Geometry: final body of the model. Coordinates: model frame, mm. Give positions to 0.01 mm unless a question says otherwise; leave off trailing zeros. Write item = value, one per line. Start each with the question number.
from build123d import *

# Parameters (mm, degrees)
CHAMFER1_SIZE                   = 3
FILLET3_R                       = 5
SKETCH3_R                       = 6
CUT_EXTRUDE3_DEPTH              = 152.492574214
CIRPATTERN2_COUNT               = 5
CIRPATTERN2_ANGLE               = 60
CIRPATTERN2_THE_OTHER_WAY_COUNT = 5
CIRPATTERN2_THE_OTHER_WAY_ANGLE = 60
MIRROR1_COPY_1_SKETCH_R         = 6
MIRROR1_COPY_1_DEPTH            = 152.492574214
MIRROR1_COPY_2_SKETCH_R         = 6
MIRROR1_COPY_2_DEPTH            = 152.492574214
MIRROR1_COPY_3_SKETCH_R         = 6
MIRROR1_COPY_3_DEPTH            = 152.492574214
MIRROR1_COPY_4_SKETCH_R         = 6
MIRROR1_COPY_4_DEPTH            = 152.492574214
MIRROR1_COPY_5_SKETCH_R         = 6
MIRROR1_COPY_5_DEPTH            = 152.492574214
MIRROR1_COPY_6_SKETCH_R         = 6
MIRROR1_COPY_6_DEPTH            = 152.492574214
MIRROR1_COPY_7_SKETCH_R         = 6
MIRROR1_COPY_7_DEPTH            = 152.492574214
MIRROR1_COPY_8_SKETCH_R         = 6
MIRROR1_COPY_8_DEPTH            = 152.492574214


with BuildPart() as part:
    # Sketch1 → Revolve1 (revolve)
    with BuildSketch(Plane.XY, mode=Mode.PRIVATE) as revolve1_sk:
        Polygon((15, 105), (7.442388155, 105), (0, 97.557611845), (-7.442388155, 105), (-15, 105), (-15, 73), (15, 73), align=None)
    revolve(revolve1_sk.sketch.rotate(Axis((0, 0, 0), (1, 0, 0)), 90), axis=Axis((0, 0, 0), (1, 0, 0)))

    # Chamfer1
    chamfer1_edges = [part.edges().sort_by_distance(p)[0] for p in [
        (15, 0, -73),
        (-15, 0, -73),
    ]]
    chamfer(chamfer1_edges, length=CHAMFER1_SIZE)

    # Fillet3
    fillet3_edges = [part.edges().sort_by_distance(p)[0] for p in [
        (0, 0, -97.557611845),
    ]]
    fillet(fillet3_edges, radius=FILLET3_R)

    # Sketch3 → Cut-Extrude3 (cut, through all)
    with BuildSketch(Plane(origin=(15, 0, 0), x_dir=(0, 0, -1), z_dir=(1, 0, 0))):
        with Locations((0, 85)):
            Circle(SKETCH3_R)
    cut_extrude3 = extrude(amount=-CUT_EXTRUDE3_DEPTH, mode=Mode.SUBTRACT)

    # CirPattern2: Cut-Extrude3 ×5 about axis
    cirpattern2_axis = Axis((0, 0, 0), (-1, 0, 0))
    for i in range(1, CIRPATTERN2_COUNT):
        add(cut_extrude3.rotate(cirpattern2_axis, i * CIRPATTERN2_ANGLE / (CIRPATTERN2_COUNT - 1)), mode=Mode.SUBTRACT)

    # CirPattern2 the other way: Cut-Extrude3 ×5 about axis
    cirpattern2_the_other_way_axis = Axis((0, 0, 0), (1, 0, 0))
    for i in range(1, CIRPATTERN2_THE_OTHER_WAY_COUNT):
        add(cut_extrude3.rotate(cirpattern2_the_other_way_axis, i * CIRPATTERN2_THE_OTHER_WAY_ANGLE / (CIRPATTERN2_THE_OTHER_WAY_COUNT - 1)), mode=Mode.SUBTRACT)

    # Mirror1: Cut-Extrude3 across plane
    add(cut_extrude3.mirror(Plane.ZX), mode=Mode.SUBTRACT)

    # Mirror1 copy 1 sketch → Mirror1 copy 1 (cut, through all)
    with BuildSketch(Plane(origin=(15, 0, 0), x_dir=(0, 0.2588190451025214, -0.9659258262890681), z_dir=(1, 0, 0))):
        with Locations((0, -85)):
            Circle(MIRROR1_COPY_1_SKETCH_R)
    extrude(amount=-MIRROR1_COPY_1_DEPTH, mode=Mode.SUBTRACT)

    # Mirror1 copy 2 sketch → Mirror1 copy 2 (cut, through all)
    with BuildSketch(Plane(origin=(15, 0, 0), x_dir=(0, 0.5000000000000011, -0.866025403784438), z_dir=(1, 0, 0))):
        with Locations((0, -85)):
            Circle(MIRROR1_COPY_2_SKETCH_R)
    extrude(amount=-MIRROR1_COPY_2_DEPTH, mode=Mode.SUBTRACT)

    # Mirror1 copy 3 sketch → Mirror1 copy 3 (cut, through all)
    with BuildSketch(Plane(origin=(15, 0, 0), x_dir=(0, 0.7071067811865488, -0.7071067811865462), z_dir=(1, 0, 0))):
        with Locations((0, -85)):
            Circle(MIRROR1_COPY_3_SKETCH_R)
    extrude(amount=-MIRROR1_COPY_3_DEPTH, mode=Mode.SUBTRACT)

    # Mirror1 copy 4 sketch → Mirror1 copy 4 (cut, through all)
    with BuildSketch(Plane(origin=(15, 0, 0), x_dir=(0, 0.8660254037844399, -0.4999999999999978), z_dir=(1, 0, 0))):
        with Locations((0, -85)):
            Circle(MIRROR1_COPY_4_SKETCH_R)
    extrude(amount=-MIRROR1_COPY_4_DEPTH, mode=Mode.SUBTRACT)

    # Mirror1 copy 5 sketch → Mirror1 copy 5 (cut, through all)
    with BuildSketch(Plane(origin=(15, 0, 0), x_dir=(0, -0.2588190451025214, -0.9659258262890681), z_dir=(1, 0, 0))):
        with Locations((0, -85)):
            Circle(MIRROR1_COPY_5_SKETCH_R)
    extrude(amount=-MIRROR1_COPY_5_DEPTH, mode=Mode.SUBTRACT)

    # Mirror1 copy 6 sketch → Mirror1 copy 6 (cut, through all)
    with BuildSketch(Plane(origin=(15, 0, 0), x_dir=(0, -0.5000000000000011, -0.866025403784438), z_dir=(1, 0, 0))):
        with Locations((0, -85)):
            Circle(MIRROR1_COPY_6_SKETCH_R)
    extrude(amount=-MIRROR1_COPY_6_DEPTH, mode=Mode.SUBTRACT)

    # Mirror1 copy 7 sketch → Mirror1 copy 7 (cut, through all)
    with BuildSketch(Plane(origin=(15, 0, 0), x_dir=(0, -0.7071067811865488, -0.7071067811865462), z_dir=(1, 0, 0))):
        with Locations((0, -85)):
            Circle(MIRROR1_COPY_7_SKETCH_R)
    extrude(amount=-MIRROR1_COPY_7_DEPTH, mode=Mode.SUBTRACT)

    # Mirror1 copy 8 sketch → Mirror1 copy 8 (cut, through all)
    with BuildSketch(Plane(origin=(15, 0, 0), x_dir=(0, -0.8660254037844399, -0.4999999999999978), z_dir=(1, 0, 0))):
        with Locations((0, -85)):
            Circle(MIRROR1_COPY_8_SKETCH_R)
    extrude(amount=-MIRROR1_COPY_8_DEPTH, mode=Mode.SUBTRACT)


solid = part.part
1) Draft query along Y for faces 1 (the cylindrical face through (11.17, -31.54, 100.15)), 2 (the cylindrical face through (0.21, 56.882, -55.043)), 3 (the flat face through (15, -70, 32)), 4 (the cylindrical face through (0.21, 76.245, -23.296)). Return one class per face: pulls with the +Y half, pulls with the -Y half, needs draft (parallel to the pull), parting line crosses it, or undercut.
2) Pin query (flat end, axial travel): pin 1 Ø1 at (x, z) = (-11, -39.5) entering from -Y; pin 2 Ø6 at (x, z) = (-11, 45.5) entering from +Y; pin 3 Ø4 at (x, y) = (-10.5, 63.5) entering from -Z. Return the tip coordinate at first contact, or that it passes through.
3) Cut plane A-A (y = 61). Give the number of separate pieces and of enclosed holes in the cut face, plus the area to 3 significant figures.
4) Ray query, L1, parallel to Z at x = 2.5, y = 78; L2, parallel to Y at x = 8.5, z = 65.5; L3, parallel to Z at x = -8.5, y = 48. Return the intervals inside material, ascending.
Reply:
q1.face_1 = parting line crosses it
q1.face_2 = undercut
q1.face_3 = needs draft
q1.face_4 = undercut
q2.pin_1 = -97.49
q2.pin_2 = 96.01
q2.pin_3 = -85.1
q3.separate_pieces = 4
q3.enclosed_holes = 0
q3.area = 1,850 mm²
q4.L1 = -63.05 to -46.59, -38.41 to -26.38, -17.62 to 17.62, 26.38 to 38.41, 46.59 to 63.05
q4.L2 = -82.07 to -62.73, -57.48 to -32.23, 32.23 to 57.48, 62.73 to 82.07
q4.L3 = -93.39 to -76.01, -71.21 to -55, 55 to 71.21, 76.01 to 93.39
